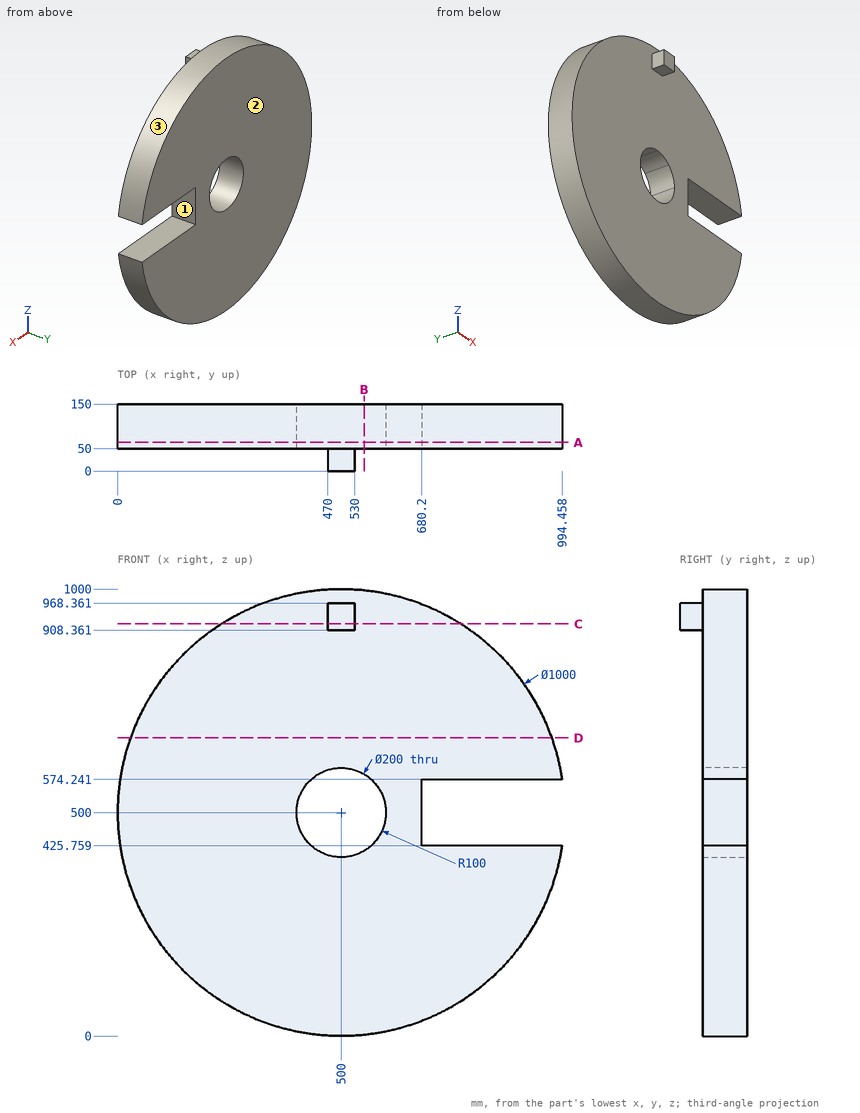
The figure shows three views and two pictorial views of one solid part (mm, origin at its lowest corner). Answer the questions. Give positions to 0.01 mm unless a question says otherwise; leave off trailing zeros. Order: outer loops, then holes, each group sorted by start corner. A loop starts at its lowest first (then second) coordinate and runs counter-clockwise, first axis right, second up. Notation, with made-up numbers: (78.5, 52) -> (107.5, 52) arc R27 ccw to (107.5, 81) -> close; hole circle Ø8 at (-13.5, -12.5). An arc over 180 degrees is marked (long way). Answer as a JSON object with one key per item and string values. Group by question number.
Item 1: The part is cut by section A-A on y = 64. Write down the section's boundary in (x, z) (1 decimal), and give its area (3 significant figures).
Item 2: The part is cut by section D-D on z = 667. Write down the section's boundary in (x, y).
Item 3: The part is cut by section B-B on x = 551.5. Write down the section's boundary in (y, z).
Item 4: Determine the mould class of the marked faces 1, 2 and 3 for opening direction Z: pulls with the +Z half, pulls with the -Z half, needs draft (parallel to the pull), parting line crosses it, or undercut.
Item 5: The part is cut by section C-C on z = 922. Write down the section's boundary in (x, y).
Item 6: Consider L1, parallel to Y at x = 355.5, z = 744; L2, parallel to Z at x = 681, y = 90.5; L3, parallel to Z at x = 685, y = 141 (1 decimal). Determine where each line is inside the solid, lowest interval first. Write a range as from..to.
Item 7: Flat-ended cylindrical pins translate along their axes: pin 1 (15 mm diameter, centred on x = 504.5, y = 26, fed in from +Z); pin 2 (1.5 mm diameter, centred on x = 828.5, z = 339, fed in from -Y); pin 3 (15 mm diameter, centred on x = 499, y = 27, fed in from -Z). Find the tip coordinate at first contact, or state that the pin passes through.
Result set:
{
 "1": {"outline": "(680.2, 425.8) -> (680.2, 574.2) -> (994.5, 574.2) arc R500 ccw (long way) to (994.5, 425.8) -> close; hole circle Ø200 at (500, 500)", "area": "707,000 mm²"},
 "2": {"outline": "(28.71, 50) -> (971.29, 50) -> (971.29, 150) -> (28.71, 150) -> close"},
 "3": {"outline": "(50, 2.66) -> (150, 2.66) -> (150, 414.28) -> (50, 414.28) -> close; (50, 585.72) -> (150, 585.72) -> (150, 997.34) -> (50, 997.34) -> close"},
 "4": {"face 1": "undercut", "face 2": "needs draft", "face 3": "parting line crosses it"},
 "5": {"outline": "(231.83, 50) -> (470, 50) -> (470, 0) -> (530, 0) -> (530, 50) -> (768.17, 50) -> (768.17, 150) -> (231.83, 150) -> close"},
 "6": {"L1": "50..150", "L2": "33.91..425.76, 574.24..966.09", "L3": "35.5..425.8, 574.2..964.5"},
 "7": {"pin 1": "z = 968.36", "pin 2": "y = 50", "pin 3": "z = 908.36"}
}
